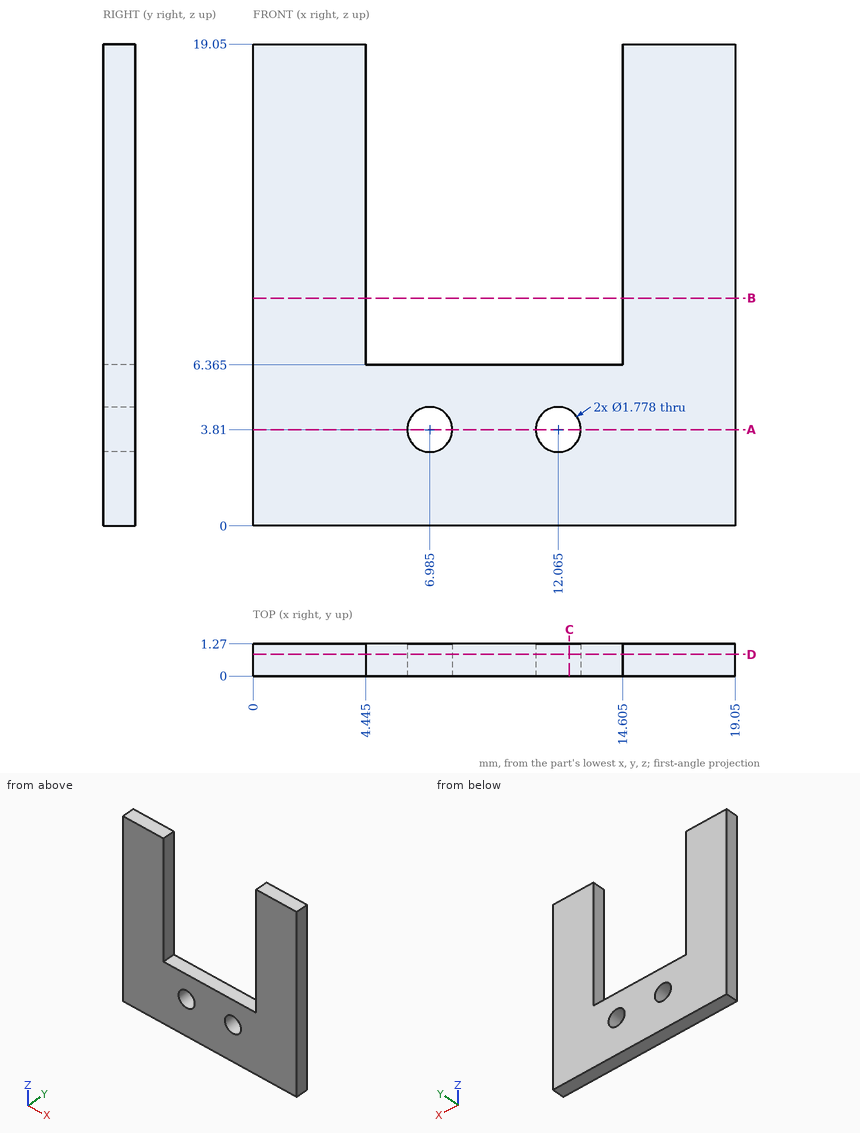
Part print with two shaded views. Sizes in mm from the minimum x, y, z corner. Coordinates: 2 decimals unless noted, no trailing zeros. Write each loop counter-clockwise with the first axis right and the second up, starting at its lowest first coordinate (ties: lowest second). Pieces come first, ordered by that corner, then holes.
(1) Cut at A-A on z = 3.81. List the corners of the cut face in (x, y), and give its area (3 significant figures).
(2) Cut at D-D on y = 0.85. List the corners of the cut face in (x, z) (3 decimals), and give its area (3 significant figures).
(3) Cut at C-C on x = 12.5. List the corners of the cut face in (y, z) (1 decimal).
(4) Drill centre lines: line 1 (X direction, y = 0.6, z = 3.81); line 2 (X direction, y = 0.55, z = 6.5) (3 decimals); line 3 (Z direction, x = 4.5, y = 1.2) (3 decimals). Where is each one in solid material? Low to high.
(5) Pin check, flat tips, straight feed: pin 1 Ø0.6 at (y, z) = (0.5, 10) entering from -X; pin 2 Ø1.1 at (x, z) = (6.985, 3.81) entering from -Y. Stop position of each tip, or through.
(6) Cut at B-B on z = 9. List the corners of the cut face in (x, y) (3 decimals), and give its area (3 significant figures).
Working result:
1. outline: (0, 0) - (6.1, 0) - (6.1, 1.27) - (0, 1.27) - close; (7.87, 0) - (11.18, 0) - (11.18, 1.27) - (7.87, 1.27) - close; (12.95, 0) - (19.05, 0) - (19.05, 1.27) - (12.95, 1.27) - close
1. area: 19.7 mm2
2. outline: (0, 0) - (19.05, 0) - (19.05, 19.05) - (14.605, 19.05) - (14.605, 6.365) - (4.445, 6.365) - (4.445, 19.05) - (0, 19.05) - close; hole circle Ø1.778 at (6.985, 3.81); hole circle Ø1.778 at (12.065, 3.81)
2. area: 229 mm2
3. outline: (0, 0) - (1.3, 0) - (1.3, 3) - (0, 3) - close; (0, 4.6) - (1.3, 4.6) - (1.3, 6.4) - (0, 6.4) - close
4. line 1: x = 0 to 6.1, 7.87 to 11.18, 12.95 to 19.05
4. line 2: x = 0 to 4.445, 14.605 to 19.05
4. line 3: z = 0 to 6.365
5. pin 1: stops at x = 0
5. pin 2: passes through
6. outline: (0, 0) - (4.445, 0) - (4.445, 1.27) - (0, 1.27) - close; (14.605, 0) - (19.05, 0) - (19.05, 1.27) - (14.605, 1.27) - close
6. area: 11.3 mm2
